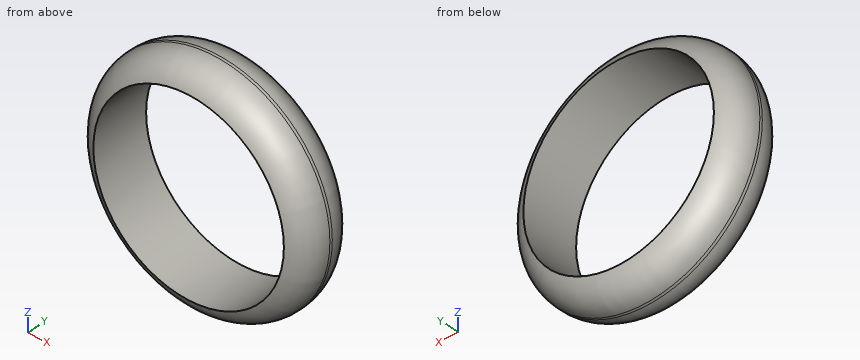
Autodesk Inventor part; units mm, degrees
ref_plane "YZ Plane" through (0, 0, 0) normal (1, 0, 0) x (0, 1, 0)
ref_plane "XZ Plane" through (0, 0, 0) normal (0, 1, 0) x (-1, 0, 0)
ref_plane "XY Plane" through (0, 0, 0) normal (0, 0, 1) x (1, 0, 0)
sketch "Boceto1" plane through (0, 0, 0) normal (0, 1, 0) x (-1, 0, 0)
  circle A0 centre (0, 0) radius 9.75
  dimension "d0" = 19.5
extrude "Extrusión1" add sketch "Boceto1" along normal blind 5
sketch "Boceto3" plane through (0, 5, 0) normal (0, 1, 0) x (1, 0, 0)
  circle A0 centre (0, 0) radius 9.75
hole "Agujero2" at (0, 5, 0) direction (0, -1, 0) diameter 16 depth 5 tip angle 118
fillet "Empalme3" radius 2.5 2 edges at (9.75, 5, 0) (9.75, 0, 0)
properties part number "exterior"
Build history of the part. All positions in model axes, mm. Round coordinates to 2 decimals unless told otherwise and drop trailing zeros. Write each loop counter-clockwise with the first axis right and the second up, starting at its lowest first coordinate (ties: lowest second). Pieces come first, ordered by that corner, then holes. Notation, with made-up numbers: (29, -19) -> (66, -19) arc R4 ccw to (66, -12) -> close; hole circle Ø10 at (77.25, 48). An arc over 180 degrees is marked (long way). Use one line per item in the form item = value.
Q1. Band-saw the part on C-C, the plane y = 1.55. Write the cut outline in (x, z), then the cut area to 3 significant figures.
Conclusion:
outline = circle Ø19.21 at (0, 0); hole circle Ø16 at (0, 0)
area = 88.9 mm²
Q2. Band-saw the part on A-A, the plane z = 0. Write the cut outline in (x, y).
Conclusion:
outline = (-9.75, 2.38) arc R2.5 ccw to (-8, 0) -> (-8, 5) arc R2.5 ccw to (-9.75, 2.62) -> close; (8, 0) arc R2.5 ccw to (9.75, 2.38) -> (9.75, 2.62) arc R2.5 ccw to (8, 5) -> close
Q3. Band-saw the part on D-D, the plane y = 4.25. Write the cut outline in (x, z).
Conclusion:
outline = circle Ø18.28 at (0, 0); hole circle Ø16 at (0, 0)
Q4. Band-saw the part on B-B, the plane x = 0. Write the cut outline in (y, z), then the cut area to 3 significant figures.
Conclusion:
outline = (0, -8) arc R2.5 ccw to (2.38, -9.75) -> (2.62, -9.75) arc R2.5 ccw to (5, -8) -> close; (0, 8) -> (5, 8) arc R2.5 ccw to (2.62, 9.75) -> (2.38, 9.75) arc R2.5 ccw to start
area = 13.1 mm²
Q5. Drill centre lines: L1, parallel to Z at x = 0, y = 1.3; L2, parallel to Z at x = 0, y = 3.9; L3, parallel to X at y = 1.5, z = 0. Where is each one in solid material? Low to high.
Conclusion:
L1 = -9.5 to -8, 8 to 9.5
L2 = -9.39 to -8, 8 to 9.39
L3 = -9.59 to -8, 8 to 9.59
Q6. Drop a flat-ended pin along its axis: P1, Ø1.5, axis at x = 6, y = 2, coming from the -Z side. Give the stop position or say it passes through.
Conclusion:
P1 = -8.19
